Read the model definition and answer for the solid it produces. Units are mm, in the model's axes. Face numbers are marked on the shaded views. A direction names the side the tool comes from. Round coordinates to 2 decimals unless told otherwise and drop trailing zeros. Loops run counter-clockwise (first coordinate to the right, second up) from the corner with the lowest first, then second, coordinate; pieces in that order, holes last. Notation, with made-up numbers: M 18.5,-37.75 L 74.5,-37.75 A22 cw 74.5,-19.75 Z; hole C -7.75,30 d6. An arc over 180 degrees is marked long. Write each question's results on one line, items separated by ' | '.
Autodesk Inventor part; units mm, degrees
ref_plane "YZ Plane" through (0, 0, 0) normal (1, 0, 0) x (0, 1, 0)
ref_plane "XZ Plane" through (0, 0, 0) normal (0, 1, 0) x (-1, 0, 0)
ref_plane "XY Plane" through (0, 0, 0) normal (0, 0, 1) x (1, 0, 0)
sketch "Sketch1" plane through (0, 0, 0) normal (1, 0, 0) x (0, 1, 0)
  line L0 (0, 0) -> (10, 0)
  line L1 (10, 0) -> (10, -10)
  line L2 (10, -10) -> (0, -10)
  line L3 (0, -10) -> (0, 0)
  dimension "d0" = 10
  dimension "d1" = 10
extrude "Extrusion1" add sketch "Sketch1" along normal blind 10
sketch "Sketch4" plane through (0, 0, 0) normal (0, 0, 1) x (1, 0, 0)
  line L0 (1.8731, 7.9408) -> (4.4271, 7.9408) construction
  line L1 (4.4271, 7.9408) -> (4.4271, 4.8928) construction
  line L2 (4.4271, 4.8928) -> (1.8731, 4.8928) construction
  line L3 (1.8731, 4.8928) -> (1.8731, 7.9408) construction
  spline S0 degree 2 poles (6.0379, 6.4263) (5.7961, 6.4263) (5.6751, 6.7102) knots 0 0 0 1 1 1
  spline S1 degree 2 poles (5.6751, 6.7102) (5.5699, 6.9521) (5.4805, 7.0047) knots 0 0 0 1 1 1
  spline S2 degree 2 poles (5.4805, 7.0047) (5.4017, 7.0468) (5.0861, 7.0468) knots 0 0 0 1 1 1
  spline S3 degree 2 poles (5.0861, 7.0468) (4.5392, 7.0468) (3.8714, 6.2107) knots 0 0 0 1 1 1
  spline S4 degree 2 poles (3.8714, 6.2107) (2.9669, 5.0853) (2.9669, 4.0809) knots 0 0 0 1 1 1
  spline S5 degree 2 poles (2.9669, 4.0809) (2.9669, 3.5919) (3.2824, 3.2448) knots 0 0 0 1 1 1
  spline S6 degree 2 poles (3.2824, 3.2448) (3.6032, 2.882) (4.0554, 2.882) knots 0 0 0 1 1 1
  spline S7 degree 2 poles (4.0554, 2.882) (4.4446, 2.882) (4.8337, 3.0818) knots 0 0 0 1 1 1
  spline S8 degree 2 poles (4.8337, 3.0818) (5.0546, 3.1975) (5.5068, 3.5288) knots 0 0 0 1 1 1
  spline S9 degree 2 poles (5.5068, 3.5288) (5.7224, 3.6865) (5.8329, 3.6865) knots 0 0 0 1 1 1
  spline S10 degree 2 poles (5.8329, 3.6865) (5.9906, 3.6865) (6.2115, 3.4394) (6.2115, 3.2921) knots 0 0 0 1 2 2 2
  spline S11 degree 2 poles (6.2115, 3.2921) (6.2115, 3.1186) (6.0695, 2.9924) knots 0 0 0 1 1 1
  spline S12 degree 2 poles (6.0695, 2.9924) (5.0704, 2.1089) (4.0554, 2.1089) knots 0 0 0 1 1 1
  spline S13 degree 2 poles (4.0554, 2.1089) (3.2719, 2.1089) (2.7355, 2.7084) knots 0 0 0 1 1 1
  spline S14 degree 2 poles (2.7355, 2.7084) (2.2149, 3.2869) (2.2149, 4.0809) knots 0 0 0 1 1 1
  spline S15 degree 2 poles (2.2149, 4.0809) (2.2149, 5.3588) (3.2877, 6.6997) knots 0 0 0 1 1 1
  spline S16 degree 2 poles (3.2877, 6.6997) (4.1817, 7.8198) (5.0861, 7.8198) knots 0 0 0 1 1 1
  spline S17 degree 2 poles (5.0861, 7.8198) (5.2702, 7.8198) (5.5647, 7.7883) (5.6804, 7.7462) knots 0 0 0 1 2 2 2
  spline S18 degree 2 poles (5.6804, 7.7462) (5.8118, 7.9408) (6.0222, 7.9408) knots 0 0 0 1 1 1
  spline S19 degree 2 poles (6.0222, 7.9408) (6.2851, 7.9408) (6.3535, 7.5989) knots 0 0 0 1 1 1
  spline S20 degree 2 poles (6.3535, 7.5989) (6.4113, 7.2887) (6.4113, 6.847) knots 0 0 0 1 1 1
  spline S21 degree 2 poles (6.4113, 6.847) (6.4113, 6.6892) (6.3272, 6.5735) knots 0 0 0 1 1 1
  spline S22 degree 2 poles (6.3272, 6.5735) (6.2273, 6.4263) (6.0379, 6.4263) knots 0 0 0 1 1 1
  point P0 (0, 0)
extrude "Extrusion4" cut sketch "Sketch4" against normal blind 2
sketch "Sketch7" plane through (0, 0, 0) normal (-1, 0, 0) x (0, 0, 1)
  line L0 (-3.1, 3.1) -> (-6.2, 3.1)
  line L1 (-6.2, 3.1) -> (-6.2, 6.2)
  line L2 (-6.2, 6.2) -> (-3.1, 6.2)
  line L3 (-3.1, 6.2) -> (-3.1, 3.1)
  point P0 (0, 0)
  dimension "d16" = 3.1
  dimension "d17" = 3.1
extrude "Extrusion6" cut sketch "Sketch7" against normal blind 5
properties part number "Cytosine1"
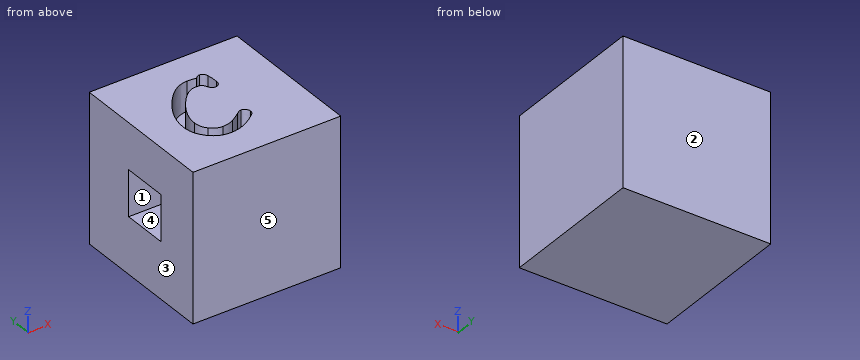
1. Find section A-A, the plane x = 0.5. Give the vertices of the cut face in (y, z).
Completed:
outline: M 0,-10 L 10,-10 L 10,0 L 0,0 Z; hole M 3.1,-6.2 L 6.2,-6.2 L 6.2,-3.1 L 3.1,-3.1 Z
2. Which of the six approach directions +Z, -Z, +X, -X, +Y, -Y give full straight-line access (tool end or side, diameter ignored) to the marked faces 4 and 5?
Completed:
face 4: -X | face 5: +Z, -Z, +X, -X, -Y
3. Find section B-B, the plane z = -5. Give the vertices of the cut face in (x, y).
Completed:
outline: M 0,0 L 10,0 L 10,10 L 0,10 L 0,6.2 L 5,6.2 L 5,3.1 L 0,3.1 Z
4. Find the intervals of material crossed by L1, parallel to Z at x = 1, y = 3.5; L2, parallel to X at y = 6.75, z = -1.75; L3, parallel to Y at x = 4.25, z = -4.25, in increasing order.
Completed:
L1: z = -10 to -6.2, -3.1 to 0 | L2: x = 0 to 3.33, 4.39 to 5.66, 6.4 to 10 | L3: y = 0 to 3.1, 6.2 to 10
5. Determine the mould class of the marked faces 1, 2 and 3 for opening direction Y: released by +Y, released by -Y, zero draft, split by the parting line, or undercut.
Completed:
face 1: undercut | face 2: released by +Y | face 3: zero draft
